Geometry: final body of the model. Coordinates: model frame, mm. A direction names the side the tool comes from. Round coordinates to 2 decimals unless told otherwise and drop trailing zeros. Write each loop counter-clockwise with the first axis right and the second up, starting at its lowest first coordinate (ties: lowest second). Pieces come first, ordered by that corner, then holes. Notation, with made-up numbers: M -2,57.5 L 15,57.5 A34 ccw 15,91.5 Z; hole C 13.25,-18.75 d8. An arc over 180 degrees is marked long. Use one line per item in the form item = value. Start each with the question number.
Item 1: Section query A-A (x = 12.5). Return loops of the section in (y, z), and give its area (3 significant figures).
Item 2: Pin query (flat end, axial travel): pin 1 Ø9 at (x, z) = (-12.5, 12.5) entering from +Y. Return the tip coordinate at first contact, or that it passes through.
Item 3: Section query B-B (z = -12.5). Return loops of the section in (x, y), and give its area (3 significant figures).
Item 4: Section query C-C (y = 4). State how many separate pieces and enclosed holes the cut face has, and give its area (3 significant figures).
Item 5: Reachability of faces 5 (the cylindrical face through (-10, 4.3, -7.6)), 6 (the flat face through (0, 4, 25)) from +Z, -Z, +X, -X, +Y, -Y: full face, straight path, thin tool, end or side. Return the list, or none.
Item 6: Pull-direction query (Z, two-part tool) for faces 1 (the flat face through (25, 4, 0)), 2 (the flat face through (21.3, 3.7, 21.2)), 3 (the cylindrical face through (17.58, 4.3, 14.61)), 4 (the flat face through (0, 4, -25)); classes: pulls with the +Z half, pulls with the -Z half, needs draft (parallel to the pull), parting line crosses it, or undercut.
Item 7: Section query D-D (x = 0). Return loops of the section in (y, z).
Item 8: Ray query, probe 1 along X at (y, z) = (0.3, -12.5); probe 2 along Z at (x, y) = (-12.5, 4); probe 3 along Z at (x, y) = (0, 2.5). Return the intervals inside material, ascending.
from build123d import *

# Parameters (mm, degrees)
SKETCH1_W                                           = 50
SKETCH1_H                                           = 50
BOSS_EXTRUDE1_DEPTH                                 = 7.5
CBORE_FOR_M6_HEX_SOCKET_HEAD_CAP_SCREW1_D           = 6.6
CBORE_FOR_M6_HEX_SOCKET_HEAD_CAP_SCREW1_DEPTH       = 7.5
CBORE_FOR_M6_HEX_SOCKET_HEAD_CAP_SCREW1_CBORE_D     = 11
CBORE_FOR_M6_HEX_SOCKET_HEAD_CAP_SCREW1_CBORE_DEPTH = 6.5
M3_TAPPED_HOLE1_D                                   = 2.5
M3_TAPPED_HOLE1_DEPTH                               = 7.5
CHAMFER1_SIZE                                       = 7.5


with BuildPart() as part:
    # Sketch1 → Boss-Extrude1 (new body)
    with BuildSketch(Plane(origin=(0, 0, 0), x_dir=(1, 0, 0), z_dir=(0, 1, 0))):
        Rectangle(SKETCH1_W, SKETCH1_H)
    extrude(amount=BOSS_EXTRUDE1_DEPTH)

    # CBORE for M6 Hex Socket Head Cap Screw1
    with Locations(Plane(origin=(0, 7.5, 0), x_dir=(1, 0, 0), z_dir=(0, 1, 0))):
        with Locations((-12.5, -12.5), (-12.5, 12.5), (12.5, 12.5), (12.5, -12.5)):
            CounterBoreHole(CBORE_FOR_M6_HEX_SOCKET_HEAD_CAP_SCREW1_D / 2, CBORE_FOR_M6_HEX_SOCKET_HEAD_CAP_SCREW1_CBORE_D / 2, CBORE_FOR_M6_HEX_SOCKET_HEAD_CAP_SCREW1_CBORE_DEPTH, depth=CBORE_FOR_M6_HEX_SOCKET_HEAD_CAP_SCREW1_DEPTH)

    # M3 Tapped Hole1
    with Locations(Plane(origin=(0, 7.5, 0), x_dir=(1, 0, 0), z_dir=(0, 1, 0))):
        with Locations((0, 17.67766953), (-17.67766953, 0), (0, -17.67766953), (17.67766953, 0)):
            Hole(M3_TAPPED_HOLE1_D / 2, depth=M3_TAPPED_HOLE1_DEPTH)

    # Chamfer1
    chamfer1_edges = [part.edges().sort_by_distance(p)[0] for p in [
        (25, 3.75, 25),
        (-25, 3.75, 25),
        (-25, 3.75, -25),
        (25, 3.75, -25),
    ]]
    chamfer(chamfer1_edges, length=CHAMFER1_SIZE)


solid = part.part
Working result:
q1.outline = M 0,-25 L 7.5,-25 L 7.5,-18 L 1,-18 L 1,-15.8 L 0,-15.8 Z; M 0,-9.2 L 1,-9.2 L 1,-7 L 7.5,-7 L 7.5,7 L 1,7 L 1,9.2 L 0,9.2 Z; M 0,15.8 L 1,15.8 L 1,18 L 7.5,18 L 7.5,25 L 0,25 Z
q1.area = 219 mm²
q2.pin_1 = 1
q3.outline = M -25,0 L -15.8,0 L -15.8,1 L -18,1 L -18,7.5 L -25,7.5 Z; M -9.2,0 L 9.2,0 L 9.2,1 L 7,1 L 7,7.5 L -7,7.5 L -7,1 L -9.2,1 Z; M 15.8,0 L 25,0 L 25,7.5 L 18,7.5 L 18,1 L 15.8,1 Z
q3.area = 219 mm²
q4.separate_pieces = 1
q4.enclosed_holes = 8
q4.area = 1,990 mm²
q5.face_5 = +Y
q5.face_6 = +Z, +X, -X, +Y, -Y
q6.face_1 = needs draft
q6.face_2 = pulls with the +Z half
q6.face_3 = undercut
q6.face_4 = pulls with the -Z half
q7.outline = M 0,-25 L 7.5,-25 L 7.5,-18.93 L 0,-18.93 Z; M 0,-16.43 L 7.5,-16.43 L 7.5,16.43 L 0,16.43 Z; M 0,18.93 L 7.5,18.93 L 7.5,25 L 0,25 Z
q8.probe_1 = -25 to -15.8, -9.2 to 9.2, 15.8 to 25
q8.probe_2 = -25 to -18, -7 to 7, 18 to 25
q8.probe_3 = -25 to -18.93, -16.43 to 16.43, 18.93 to 25
